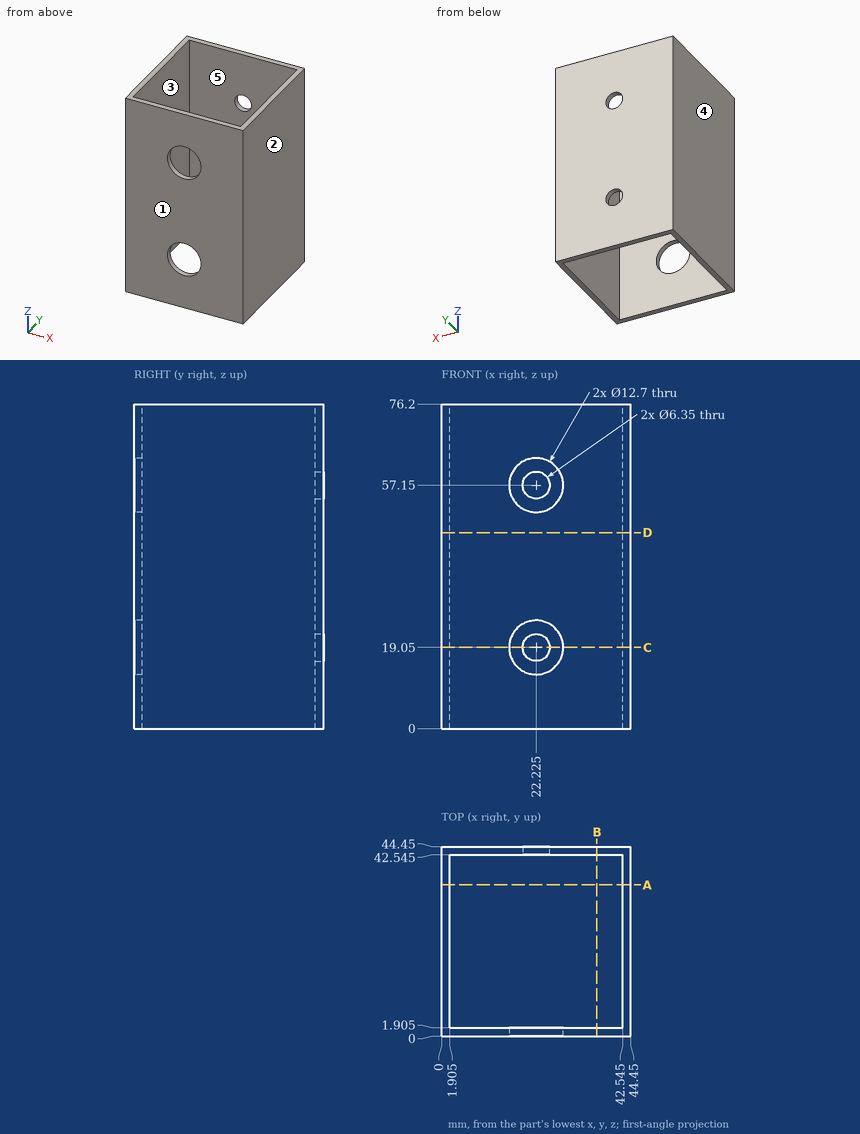
The drawing under review shows one solid part. Ordinate dimensions are in mm from its lowest x, y, z. A direction names the side the tool comes from. Give positions to 0.01 mm unless a question says otherwise; leave off trailing zeros. Loops run counter-clockwise (first coordinate to the right, second up) from the corner with the lowest first, then second, coordinate; pieces in that order, holes last. Notation, with made-up numbers: M 42,-19.75 L 51,-19.75 A11 ccw 51,-8.75 Z; hole C 74,-27 d9. An arc over 180 degrees is marked long. One line per item, written item: value. Start each with the question number.
Q1. Machinability: for the marked faces 4 and 5, which of the approach directions +Z, -Z, +X, -X, +Y, -Y give a long, thin tool a straight path to every point of the face, cutting with its end or side? Answer none if there is none.
Q2. Add section A-A (y = 35.5). Give the boundary of the cut face in (x, z) (3 decimals).
Q3. For L1, parallel to Y at x = 28, z = 45.5 (3 decimals); L2, parallel to X at y = 44, z = 57, list the stretches that pass through material, from the lowest coordinate up.
Q4. Clearance check with a flat-ended pin moving along its axis: pin 1 Ø8.5 at (x, z) = (22.225, 57.15) entering from -Y (3 decimals). State where the tip first meets the part, or that it passes through.
Q5. Add section D-D (z = 46). Give the boundary of the cut face in (x, y) (3 decimals).
Q6. Draft analysis for pull direction X (two halves, no side actions). For the marked faces 1, 2 and 3, state which applies: released by +X, released by -X, zero draft, split by the parting line, or undercut.
Q7. Add section C-C (z = 19.05). Give the boundary of the cut face in (x, y) (3 decimals), and give its area (3 significant figures).
Reply:
1. face 4: +Z, -Z, -X, +Y, -Y
1. face 5: +Z, -Z
2. outline: M 0,0 L 1.905,0 L 1.905,76.2 L 0,76.2 Z; M 42.545,0 L 44.45,0 L 44.45,76.2 L 42.545,76.2 Z
3. L1: 0 to 1.905, 42.545 to 44.45
3. L2: 0 to 19.05, 25.4 to 44.45
4. pin 1: y = 42.545
5. outline: M 0,0 L 44.45,0 L 44.45,44.45 L 0,44.45 Z; hole M 1.905,1.905 L 42.545,1.905 L 42.545,42.545 L 1.905,42.545 Z
6. face 1: zero draft
6. face 2: released by +X
6. face 3: undercut
7. outline: M 0,0 L 15.875,0 L 15.875,1.905 L 1.905,1.905 L 1.905,42.545 L 19.05,42.545 L 19.05,44.45 L 0,44.45 Z; M 25.4,42.545 L 42.545,42.545 L 42.545,1.905 L 28.575,1.905 L 28.575,0 L 44.45,0 L 44.45,44.45 L 25.4,44.45 Z
7. area: 288 mm²
